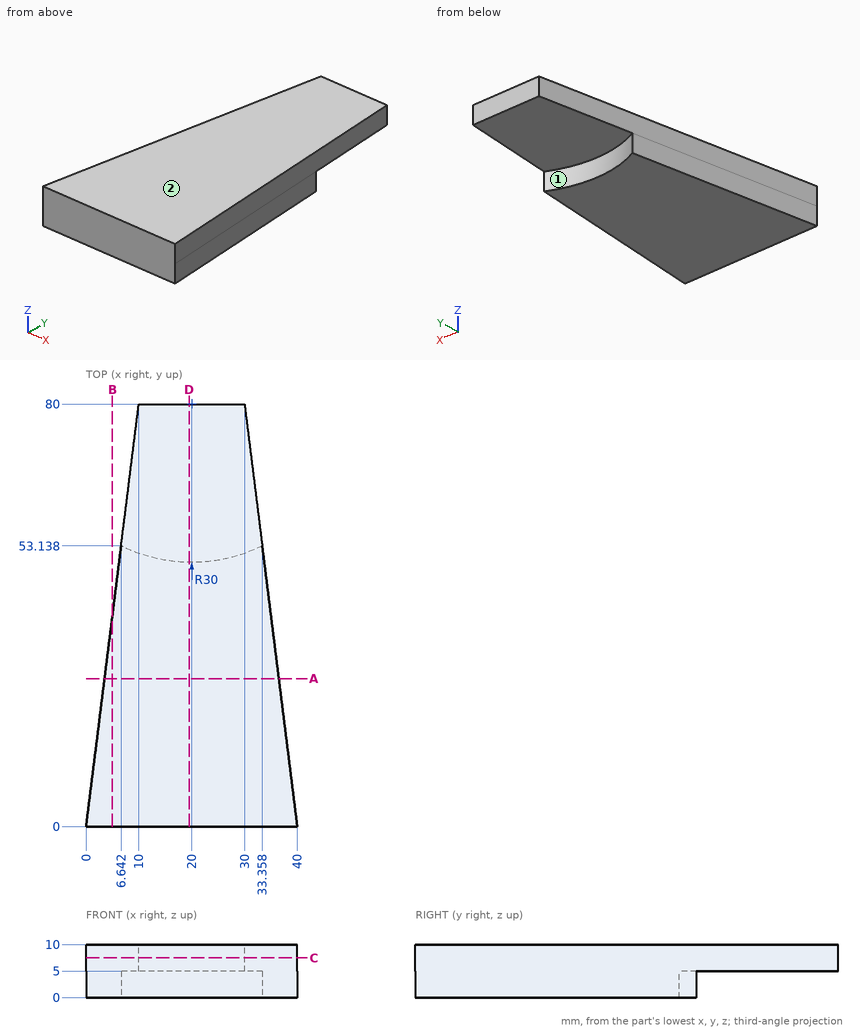
The figure shows three views and two pictorial views of one solid part (mm, origin at its lowest corner). Answer the questions. Give positions to 0.01 mm unless a question says otherwise; leave off trailing zeros. Loops run counter-clockwise (first coordinate to the right, second up) from the corner with the lowest first, then second, coordinate; pieces in that order, holes last. Notation, with made-up numbers: (-11.5, -4.5) -> (18.5, -4.5) arc R19 ccw to (18.5, 26.5) -> close; hole circle Ø7 at (9.25, -5). An arc over 180 degrees is marked (long way). Put each result on its own line as item: value. Start each with the question number.
Item 1: The part is cut by section D-D (x = 19.5). Give the vertices of the cut face in (y, z), then the cut area to 3 significant figures.
Item 2: Find the intervals of material crossed by L1, parallel to Z at x = 17.5, y = 62.5; L2, parallel to X at y = 51, z = 9 (1 decimal); L3, parallel to Y at x = 22, z = 3.25, in increasing order. Write a range as [from, to].
Item 3: The part is cut by section B-B (x = 5). Give the vertices of the cut face in (y, z).
Item 4: The part is cut by section C-C (z = 7.5). Give the vertices of the cut face in (x, y), then the cut area to 3 significant figures.
Item 5: The mould has two halves that part along X. Classify the marked faces 1 and 2: released by +X, released by -X, zero draft, split by the parting line, or undercut.
Item 6: The part is cut by section A-A (y = 28). Give the vertices of the cut face in (x, z), then the cut area to 3 significant figures.
Item 7: Each of these flat-tipped pins is pushed along its axis until it touches: P1, Ø6, axis at y = 67, z = 3.5, coming from the +X side; P2, Ø13.5, axis at x = 26, y = 67, coming from the -Z side. Where does it stop, or does it pass through?
Answers below:
1. outline: (0, 0) -> (50, 0) -> (50, 5) -> (80, 5) -> (80, 10) -> (0, 10) -> close
1. area: 650 mm2
2. L1: [5, 10]
2. L2: [6.4, 33.6]
2. L3: [0, 50.07]
3. outline: (0, 0) -> (40, 0) -> (40, 10) -> (0, 10) -> close
4. outline: (0, 0) -> (40, 0) -> (30, 80) -> (10, 80) -> close
4. area: 2,400 mm2
5. face 1: undercut
5. face 2: zero draft
6. outline: (3.5, 0) -> (36.5, 0) -> (36.5, 10) -> (3.5, 10) -> close
6. area: 330 mm2
7. P1: x = 31.95
7. P2: z = 5
